from build123d import *

# Parameters (mm, degrees)
F0_R     = 101.6
F0_R_2   = 50.8
F1_DEPTH = 74.6125
F2_R     = 5.08
F3_SIZE  = 5.08


with BuildPart() as f1:
    # F0 (on Front) → F1 (new body, symmetric)
    with BuildSketch(Plane.XZ):
        with Locations((0, 9.641961284)):
            Circle(F0_R)
        with Locations((0, 9.641961284)):
            Circle(F0_R_2, mode=Mode.SUBTRACT)
    extrude(amount=F1_DEPTH, both=True)

    # F2
    f2_edges = [f1.edges().sort_by_distance(p)[0] for p in [
        (-101.6, 74.6125, 9.641961),
        (101.6, 0, 9.641961),
        (-101.6, -74.6125, 9.641961),
    ]]
    fillet(f2_edges, radius=F2_R)

    # F3
    f3_edges = [f1.edges().sort_by_distance(p)[0] for p in [
        (-50.8, -74.6125, 9.641961),
        (50.8, 0, 9.641961),
        (-50.8, 74.6125, 9.641961),
    ]]
    chamfer(f3_edges, length=F3_SIZE)


solid = f1.part
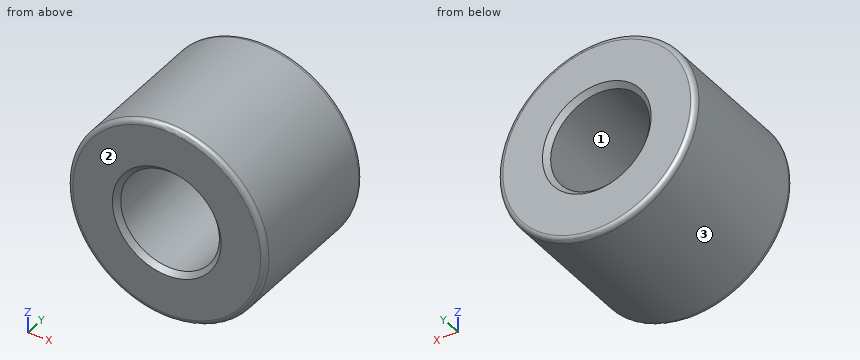
Here's how the part is built. I have some questions about the finished solid (model axes, mm). Face numbers are marked on the shaded views. Coordinates: 2 decimals unless noted, no trailing zeros. Loops run counter-clockwise (first coordinate to the right, second up) from the corner with the lowest first, then second, coordinate; pieces in that order, holes last. Notation, with made-up numbers: (84.5, 56) -> (136.5, 56) arc R21 ccw to (136.5, 88) -> close; hole circle Ø5 at (-9.75, 64.5). An arc over 180 degrees is marked (long way). Use one line per item in the form item = value. Start each with the question number.
(1) Will these pins go through, and if not, where does the flat tip stop? pin 1 (12 mm diameter, centred on x = 30.5, y = -49.5, fed in from -Z); pin 2 (2 mm diameter, centred on x = -54.5, y = 32.5, fed in from +Z); pin 3 (6 mm diameter, centred on y = -45, z = -37.5, fed in from -X).
(2) Please list where these lines run through material, in increasing order: line 1 along Z through (x, y) = (0, -4); line 2 along Z through (x, y) = (-7.5, 22); line 3 along X through (y, z) = (53, 16).
(3) We'd pull the mould along X, two halves only. Please class the marked faces 1, 2 and 3: pulls with the +X half, pulls with the -X half, needs draft (parallel to the pull), parting line crosses it, or undercut.
(4) If we section it at B-B (y = 51.5): Please give me the cut outline in (x, z), then the cut area to 3 significant figures.
(5) If we section it at A-A (x = 0): Please give me the cut outline in (y, z).
Verdict:
q1.pin_1 = -88.96
q1.pin_2 = 96.02
q1.pin_3 = -91.51
q2.line_1 = -91.96 to -41.16, 60.44 to 111.24
q2.line_2 = -91.68 to -40.6, 59.89 to 110.96
q2.line_3 = -101.4 to -50.4, 50.4 to 101.4
q3.face_1 = undercut
q3.face_2 = needs draft
q3.face_3 = parting line crosses it
q4.outline = circle Ø203.2 at (0, 9.64); hole circle Ø101.6 at (0, 9.64)
q4.area = 24,300 mm²
q5.outline = (-74.61, -86.88) arc R5.08 ccw to (-69.53, -91.96) -> (69.53, -91.96) arc R5.08 ccw to (74.61, -86.88) -> (74.61, -46.24) -> (69.53, -41.16) -> (-69.53, -41.16) -> (-74.61, -46.24) -> close; (-74.61, 65.52) -> (-69.53, 60.44) -> (69.53, 60.44) -> (74.61, 65.52) -> (74.61, 106.16) arc R5.08 ccw to (69.53, 111.24) -> (-69.53, 111.24) arc R5.08 ccw to (-74.61, 106.16) -> close
